from build123d import *

# Parameters (mm, degrees)
SKETCH1_W           = 80
SKETCH1_H           = 15
BOSS_EXTRUDE1_DEPTH = 6
CUT_EXTRUDE1_DEPTH  = 82.614949611
SKETCH3_W           = 25
SKETCH3_H           = 12
CUT_EXTRUDE2_DEPTH  = 82.614949611
SKETCH4_W           = 4
SKETCH4_H           = 1.5
BOSS_EXTRUDE2_DEPTH = 2
SKETCH5_W           = 4
SKETCH5_H           = 1.5
BOSS_EXTRUDE3_DEPTH = 2
SKETCH6_W           = 4
SKETCH6_H           = 1.5
BOSS_EXTRUDE4_DEPTH = 2
SKETCH7_W           = 4
SKETCH7_H           = 1.5
BOSS_EXTRUDE5_DEPTH = 2
SKETCH9_W           = 4
SKETCH9_H           = 1.5
BOSS_EXTRUDE6_DEPTH = 2
SKETCH10_W          = 4
SKETCH10_H          = 1.5
BOSS_EXTRUDE7_DEPTH = 2
SKETCH12_W          = 4
SKETCH12_H          = 1.5
BOSS_EXTRUDE8_DEPTH = 2
SKETCH12_3_W        = 4
SKETCH12_3_H        = 1.5
BOSS_EXTRUDE9_DEPTH = 2


with BuildPart() as part:
    # Sketch1 → Boss-Extrude1 (new body)
    with BuildSketch(Plane.XY):
        with Locations((40, 7.5)):
            Rectangle(SKETCH1_W, SKETCH1_H)
    extrude(amount=BOSS_EXTRUDE1_DEPTH)

    # Sketch2 → Cut-Extrude1 (cut, through all)
    with BuildSketch(Plane(origin=(0, 15, 0), x_dir=(1, 0, 0), z_dir=(0, 1, 0))):
        Polygon((74, 0), (74, -2), (77, -2), (77, -4), (71, -4), (71, 0), align=None)
    extrude(amount=-CUT_EXTRUDE1_DEPTH, mode=Mode.SUBTRACT)

    # Sketch3 → Cut-Extrude2 (cut, through all)
    with BuildSketch(Plane.XY.offset(6)):
        with Locations((15, 7.5)):
            Rectangle(SKETCH3_W, SKETCH3_H)
    extrude(amount=-CUT_EXTRUDE2_DEPTH, mode=Mode.SUBTRACT)

    # Sketch4 → Boss-Extrude2 (add)
    with BuildSketch(Plane.XY.offset(6)):
        with Locations((4.5, 14.25)):
            Rectangle(SKETCH4_W, SKETCH4_H)
    extrude(amount=BOSS_EXTRUDE2_DEPTH)

    # Sketch5 → Boss-Extrude3 (add)
    with BuildSketch(Plane.XY.offset(6)):
        with Locations((14.5, 14.25)):
            Rectangle(SKETCH5_W, SKETCH5_H)
    extrude(amount=BOSS_EXTRUDE3_DEPTH)

    # Sketch6 → Boss-Extrude4 (add)
    with BuildSketch(Plane.XY.offset(6)):
        with Locations((4.5, 0.75)):
            Rectangle(SKETCH6_W, SKETCH6_H)
    extrude(amount=BOSS_EXTRUDE4_DEPTH)

    # Sketch7 → Boss-Extrude5 (add)
    with BuildSketch(Plane.XY.offset(6)):
        with Locations((14.5, 0.75)):
            Rectangle(SKETCH7_W, SKETCH7_H)
    extrude(amount=BOSS_EXTRUDE5_DEPTH)

    # Sketch9 → Boss-Extrude6 (add)
    with BuildSketch(Plane(origin=(0, 0, 0), x_dir=(-1, 0, 0), z_dir=(0, 0, -1))):
        with Locations((-4.5, 14.25)):
            Rectangle(SKETCH9_W, SKETCH9_H)
    extrude(amount=BOSS_EXTRUDE6_DEPTH)

    # Sketch10 → Boss-Extrude7 (add)
    with BuildSketch(Plane(origin=(0, 0, 0), x_dir=(-1, 0, 0), z_dir=(0, 0, -1))):
        with Locations((-14.5, 14.25)):
            Rectangle(SKETCH10_W, SKETCH10_H)
    extrude(amount=BOSS_EXTRUDE7_DEPTH)

    # Sketch12 → Boss-Extrude8 (add)
    with BuildSketch(Plane(origin=(0, 0, 0), x_dir=(-1, 0, 0), z_dir=(0, 0, -1))):
        with Locations((-14.5, 0.75)):
            Rectangle(SKETCH12_W, SKETCH12_H)
    extrude(amount=BOSS_EXTRUDE8_DEPTH)

    # Sketch12<3> → Boss-Extrude9 (add)
    with BuildSketch(Plane(origin=(0, 0, 0), x_dir=(-1, 0, 0), z_dir=(0, 0, -1))):
        with Locations((-4.5, 0.75)):
            Rectangle(SKETCH12_3_W, SKETCH12_3_H)
        with Locations((-14.5, 0.75)):
            Rectangle(SKETCH12_3_W, SKETCH12_3_H)
    extrude(amount=BOSS_EXTRUDE9_DEPTH)


solid = part.part
The listing builds one solid part. Answer for the finished solid, in the listing's coordinates (mm). A direction names the side the tool comes from. Give positions to 0.01 mm unless a question says otherwise; leave off trailing zeros. Write each loop counter-clockwise with the first axis right and the second up, starting at its lowest first coordinate (ties: lowest second). Pieces come first, ordered by that corner, then holes. Notation, with made-up numbers: (43, 14) -> (84, 14) arc R14 cw to (84, 32) -> close; hole circle Ø8 at (25.5, -5.5). An arc over 180 degrees is marked (long way). Use a Markdown table: item, result.
(1) For faces 5 (the flat face through (16.5, 1, 7)), 6 (the flat face through (6.5, 14, -1)), 7 (the flat face through (1, 8, 6)), 8 (the flat face through (12.5, 14, 7)), determine the directions among +Z, -Z, +X, -X, +Y, -Y from which every point of the face is accessible in a straight line to the end or side of a thin tool.
Return value:
| item | result |
|---|---|
| face 5 | +Z, +X, +Y, -Y |
| face 6 | -Z, +Y, -Y |
| face 7 | +Z, -X, +Y, -Y |
| face 8 | +Z, +Y, -Y |
(2) Find the intervals of material crossed by probe 1 along X at (y, z) = (4, 0.75); probe 2 along X at (y, z) = (4, 5.25); probe 3 along Y at (x, z) = (15, 2.75), in increasing order. Write a range as from..to.
Return value:
| item | result |
|---|---|
| probe 1 | 0..2.5, 27.5..71, 74..80 |
| probe 2 | 0..2.5, 27.5..80 |
| probe 3 | 0..1.5, 13.5..15 |
(3) Section D-D, the plane z = 7.25 is taken. Determine the outline of the cut face in (x, y), then the cut area to 3 significant figures.
Return value:
| item | result |
|---|---|
| outline | (2.5, 0) -> (6.5, 0) -> (6.5, 1.5) -> (2.5, 1.5) -> close; (2.5, 13.5) -> (6.5, 13.5) -> (6.5, 15) -> (2.5, 15) -> close; (12.5, 0) -> (16.5, 0) -> (16.5, 1.5) -> (12.5, 1.5) -> close; (12.5, 13.5) -> (16.5, 13.5) -> (16.5, 15) -> (12.5, 15) -> close |
| area | 24.0 mm2 |
(4) Flat-ended cylindrical pins translate along their axes: P1, Ø3, axis at x = 17, z = 7, coming from the -Y side; P2, Ø1.6, axis at y = 0.5, z = -1.5, coming from the +X side; P3, Ø1, axis at x = 59, y = 9, coming from the +Z side; P4, Ø2, axis at x = 55, y = 6, coming from the -Z side. Find the tip coordinate at first contact, or state that the pin passes through.
Return value:
| item | result |
|---|---|
| P1 | y = 0 |
| P2 | x = 16.5 |
| P3 | z = 6 |
| P4 | z = 0 |
(5) Section C-C, the plane y = 8 is taken. Determine the outline of the cut face in (x, z).
Return value:
| item | result |
|---|---|
| outline | (0, 0) -> (2.5, 0) -> (2.5, 6) -> (0, 6) -> close; (27.5, 0) -> (71, 0) -> (71, 4) -> (77, 4) -> (77, 2) -> (74, 2) -> (74, 0) -> (80, 0) -> (80, 6) -> (27.5, 6) -> close |
(6) Section A-A, the plane z = 3.25 is taken. Determine the outline of the cut face in (x, y).
Return value:
| item | result |
|---|---|
| outline | (0, 0) -> (71, 0) -> (71, 15) -> (0, 15) -> close; (77, 0) -> (80, 0) -> (80, 15) -> (77, 15) -> close; hole (2.5, 1.5) -> (27.5, 1.5) -> (27.5, 13.5) -> (2.5, 13.5) -> close |
(7) Determine the mould class of faces 1 (the flat face through (9, 1, 0)), 2 (the flat face through (2.5, 14, 7)), 3 (the flat face through (74, 8, 4)), 4 (the flat face through (77, 8, 3)) for opening direction Z: released by +Z, released by -Z, zero draft, split by the parting line, or undercut.
Return value:
| item | result |
|---|---|
| face 1 | released by -Z |
| face 2 | zero draft |
| face 3 | undercut |
| face 4 | undercut |
(8) Section B-B, the plane x = 20 is taken. Determine the outline of the cut face in (y, z), then the cut area to 3 significant figures.
Return value:
| item | result |
|---|---|
| outline | (0, 0) -> (1.5, 0) -> (1.5, 6) -> (0, 6) -> close; (13.5, 0) -> (15, 0) -> (15, 6) -> (13.5, 6) -> close |
| area | 18.0 mm2 |
